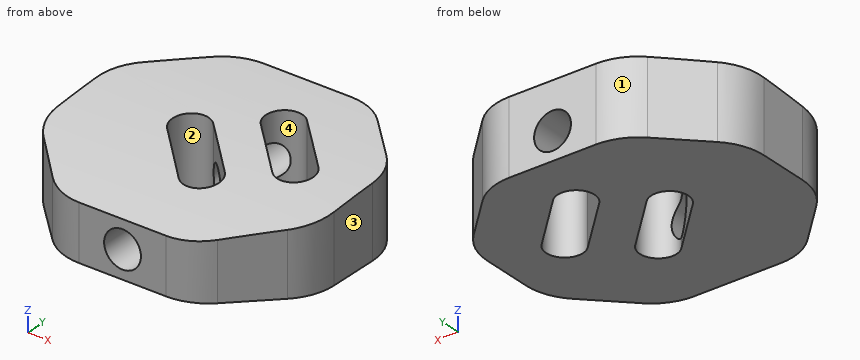
Autodesk Inventor part; units mm, degrees
ref_plane "YZ Plane" through (0, 0, 0) normal (1, 0, 0) x (0, 1, 0)
ref_plane "XZ Plane" through (0, 0, 0) normal (0, 1, 0) x (-1, 0, 0)
ref_plane "XY Plane" through (0, 0, 0) normal (0, 0, 1) x (1, 0, 0)
sketch "Base" plane through (0, 0, 0) normal (0, 0, 1) x (1, 0, 0)
  line L0 (-7.5, -2.6) -> (-7.5, 2.6)
  line L1 (-7.5, 2.6) -> (-3.6, 6.5)
  line L2 (-3.6, 6.5) -> (3.6, 6.5)
  line L3 (3.6, 6.5) -> (7.5, 2.6)
  line L4 (7.5, 2.6) -> (7.5, -2.6)
  line L5 (7.5, -2.6) -> (3.6, -6.5)
  line L6 (3.6, -6.5) -> (-3.6, -6.5)
  line L7 (-3.6, -6.5) -> (-7.5, -2.6)
  line L8 (-7.5, 0) -> (7.5, 0) construction
  line L9 (0, 6.5) -> (0, -6.5) construction
  point P0 (0, 0)
  point P1 (0, 0)
  dimension "d1" = 15
  dimension "d5" = 13
  dimension "d7" = 5.2
extrude "BaseFeature" add sketch "Base" along normal blind 4
fillet "BaseFilletsFeature" radius 3 8 edges at (-7.5, -2.6, 2) (-3.6, -6.5, 2) (3.6, -6.5, 2) (7.5, -2.6, 2) (7.5, 2.6, 2) (3.6, 6.5, 2) (-3.6, 6.5, 2) (-7.5, 2.6, 2)
sketch "RailHoles" plane through (0, 0, 4) normal (0, 0, 1) x (1, 0, 0)
  line L0 (1.3503, 3.0929) -> (4.0929, 0.3503) construction
  line L1 (-1.7888, 0.5751) -> (0.9538, -2.1675) construction
  line L2 (6.6213, 3.4787) -> (4.4787, 5.6213) construction
  line L3 (5.55, 4.55) -> (2.7216, 1.7216) construction
  circle A0 centre (1.3503, 3.0929) radius 1
  circle A1 centre (4.0929, 0.3503) radius 1
  circle A2 centre (-1.7888, 0.5751) radius 1
  circle A3 centre (0.9538, -2.1675) radius 1
  line L4 (2.0574, 3.8) -> (4.8, 1.0574)
  line L5 (0.6432, 2.3858) -> (3.3858, -0.3568)
  line L6 (-1.0817, 1.2822) -> (1.6609, -1.4604)
  line L7 (-2.4959, -0.132) -> (0.2467, -2.8746)
  dimension "d11" = 4
  dimension "d12" = 4
  dimension "d13" = 3.8786
  dimension "d14" = 2
  dimension "d15" = 1.5
  dimension "d25" = 3.0301
extrude "RailHolesFeature" cut sketch "RailHoles" against normal through all
sketch "RouteHole" plane through (-2.3574, -6.5, 0) normal (0, -1, 0) x (1, 0, 0)
  line L0 (4.7147, 4) -> (4.7147, 0) construction
  line L1 (0, 4) -> (4.7147, 4) construction
  line L2 (0, 0) -> (0, 4) construction
  line L3 (4.7147, 0) -> (0, 0) construction
  line L4 (0, 4) -> (0, 0) construction
  line L5 (0, 4) -> (4.7147, 4) construction
  line L6 (2.3574, 4) -> (2.3574, 0) construction
  line L7 (4.7147, 0) -> (0, 0) construction
  circle A0 centre (2.3574, 1.5) radius 1.25
  dimension "d40" = 2.5
  dimension "d41" = 1.5
hole "RouteHoleFeature" at (0, -6.5, 1.5) direction (0, 1, 0) diameter 2 end through all
sketch "SideProfile" plane through (7.5, -1.3574, 0) normal (1, 0, 0) x (0, 0, -1)
  arc A0 (-4, 7.8574) -> (-3, -5.1426) centre (81, 7.8574) ccw
  line L0 (-4, -5.1426) -> (0, -5.1426) construction
  line L1 (0, 7.8574) -> (-4, 7.8574) construction
  line L2 (-3, -5.1426) -> (0, -5.1426)
  line L3 (0, 7.8574) -> (0, -5.1426)
  line L4 (0, 7.8574) -> (0, 6.9787)
  line L5 (0, 7.8574) -> (-4, 7.8574)
  line L6 (-4, -2.1213) -> (-4, 0) construction
  dimension "d36" = 4
  dimension "d39" = 3
extrude "SideProfileFeature" cut sketch "SideProfile" against normal through all keep common part
equation "\"d7\" = 0.4 * d5"
equation "\"d12\" = 2 * d14"
equation "\"d13\" = 1.28 * d25"
properties part number "RingRouter"
Model file for the job. Use its own axes, mm. Face numbers are marked on the shaded views. Coordinates: 2 decimals unless noted, no trailing zeros. Loops run counter-clockwise (first coordinate to the right, second up) from the corner with the lowest first, then second, coordinate; pieces in that order, holes last. Notation, with made-up numbers: (16.5, 50) - (73.5, 50) arc R15 ccw to (73.5, 68) - close; hole circle Ø1 at (-13.75, 26.25). An arc over 180 degrees is marked (long way). Answer as a JSON object with one key per item and string values. Group by question number.
(1) Flat gauge pin, fed straight in: pin 1 (1 mm diameter, centred on x = -5, z = 1.5, fed in from -Y). Where does the tip first touch, or does it go through?
(2) Cut at D-D (x = 0). Give the cut face in (y, z).
(3) Probe line 1 along Z through (x, y) = (0, 1.25); line 2 along X through (y, z) = (-3.45, 1.5); line 3 along Z through (x, y) = (-1.75, 6). List the from-to ranges inside material, lowest first.
(4) Two-plate mould, pull along Y, no slides. Class the marked faces 1, 2, 3 and 4: released by +Y, released by -Y, zero draft, split by the parting line, or undercut.
(5) Cut at C-C (x = -1.75). Give the cut face in (y, z).
(6) Cut at A-A (y = 1.75). Give the cut face in (x, z), then the cut area to 3 significant figures.
Geometry says:
{
 "1": {"pin 1": "stops at y = -5.6"},
 "2": {"outline": "(-6.5, 0) - (-2.63, 0) - (-2.63, 0.5) - (-6.5, 0.5) - close; (-6.5, 2.5) - (-2.63, 2.5) - (-2.63, 3.51) arc R85 ccw to (-6.5, 3) - close; (0.2, 0) - (6.5, 0) - (6.5, 0.5) - (0.2, 0.5) - close; (0.2, 2.5) - (6.5, 2.5) - (6.5, 4) arc R85 ccw to (0.2, 3.77) - close"},
 "3": {"line 1": "z = 0 to 0.5, 2.5 to 3.84", "line 2": "x = -6.65 to -1, 1 to 6.65", "line 3": "z = 0 to 4"},
 "4": {"face 1": "released by +Y", "face 2": "undercut", "face 3": "zero draft", "face 4": "undercut"},
 "5": {"outline": "(-6.5, 0) - (-0.88, 0) - (-0.88, 3.68) arc R85 ccw to (-6.5, 3) - close; (1.57, 0) - (6.5, 0) - (6.5, 4) arc R85 ccw to (1.57, 3.86) - close"},
 "6": {"outline": "(-7.47, 0) - (1.28, 0) - (1.28, 3.87) - (-7.47, 3.87) - close; (4.11, 0) - (7.47, 0) - (7.47, 3.87) - (4.11, 3.87) - close; hole circle Ø2 at (0, 1.5)", "area": "43.7 mm^2"}
}
